```python
from build123d import *

# Parameters (mm, degrees)
F0_R     = 12.7
F1_DEPTH = 44.45
F2_W     = 127
F2_H     = 67.31
F3_DEPTH = 12.7
F4_R     = 5.08
F5_DEPTH = 13.7612578348


with BuildPart() as f1:
    # F0 (on Front) → F1 (new body)
    with BuildSketch(Plane.XZ):
        with BuildLine():
            Line((-31.75, 12.7), (-31.75, 0))
            Line((-31.75, 0), (31.75, 0))
            Line((31.75, 0), (31.75, 12.7))
            Line((31.75, 12.7), (12.7, 12.7))
            Line((12.7, 12.7), (12.7, 21.59))
            Line((12.7, 21.59), (63.5, 21.59))
            Line((63.5, 21.59), (63.5, 34.29))
            Line((63.5, 34.29), (47.625, 34.29))
            Line((47.625, 34.29), (21.6717633531, 76.7474402496))
            ThreePointArc((21.6717633531, 76.7474402496), (0, 88.9), (-21.6717633531, 76.7474402496))
            Line((-21.6717633531, 76.7474402496), (-47.625, 34.29))
            Line((-47.625, 34.29), (-63.5, 34.29))
            Line((-63.5, 34.29), (-63.5, 21.59))
            Line((-63.5, 21.59), (-12.7, 21.59))
            Line((-12.7, 21.59), (-12.7, 12.7))
            Line((-12.7, 12.7), (-31.75, 12.7))
        make_face()
        with Locations((0, 63.5)):
            Circle(F0_R, mode=Mode.SUBTRACT)
    extrude(amount=F1_DEPTH)

    # F2 (on face) → F3 (join)
    with BuildSketch(Plane(origin=(0, 0, 0), x_dir=(-1, 0, 0), z_dir=(0, 1, 0))):
        with Locations((0, 55.245)):
            Rectangle(F2_W, F2_H)
        Polygon((12.7, 21.59), (-12.7, 21.59), (-12.7, 12.7), (-31.75, 12.7), (-31.75, 0), (31.75, 0), (31.75, 12.7), (12.7, 12.7), align=None)
    extrude(amount=F3_DEPTH)

    # F4 (on face) → F5 (cut, through all)
    with BuildSketch(Plane.XY.offset(88.9)):
        with Locations((0, -22.225)):
            Circle(F4_R)
    extrude(amount=-F5_DEPTH, mode=Mode.SUBTRACT)


solid = f1.part
```
Source: CAD feature listing. Evaluate the final solid. Frame: model axes, mm. A direction names the side the tool comes from. Coordinates: 2 decimals unless noted, no trailing zeros. Order: outer loops, then holes, each group sorted by start corner. A loop starts at its lowest first (then second) coordinate and runs counter-clockwise, first axis right, second up. Notation, with made-up numbers: M -36.75,9 L 18.25,9 A26 ccw 18.25,43 Z; hole C 47.5,73.25 d3. An arc over 180 degrees is marked long. Write each question's results on one line, items separated by ' | '. Start each with the question number.
1) Section query A-A (y = -34). Return the cut outline in (x, z) (3 decimals), plus the area to 3 significant figures.
2) Draft query along X for faces 6 (the face through (1, 12.7, 55)), 7 (the face through (5.86, -21.914, 52.233)), 8 (the face through (0.363, -16.975, 88.897)). Return one class per face: released by +X, released by -X, zero draft, split by the parting line, or undercut.
3) Contact query for flat-ended pins moving along their axis: pin 1 Ø1.5 at (x, y) = (47, 0) entering from -Z; pin 2 Ø6.5 at (y, z) = (-18.5, 6) entering from +X; pin 3 Ø15 at (x, y) = (-24.5, -27.5) entering from +Z. Output: stop coordinate, or through.
4) Section query D-D (x = 55). Return the cut outline in (y, z).
5) Section query B-B (x = 20). Return the cut outline in (y, z), plus the area to 3 significant figures.
6) Line query: line 1 (Z direction, x = 0, y = -10.5); line 2 (Y direction, x = 0, z = 80.75) (3 decimals); line 3 (Y direction, x = -53.5, z = 60.5). Output: solid intervals per line, ascending. Write a range as from..to.
7) Access query for faces 1 (the face through (46, 0, 68)), 2 (the face through (0, 0, 64)), 3 (the face through (-38, -16, 21.59)), 4 (the face through (-34.467, -21.914, 55.816)), 5 (the face through (-31.75, -16, 6)). Directions: +Z, -Z, +X, -X, +Y, -Y. A direction counts if a zero-diameter tool reaches every point of the face in a straight line with its end or side. Return the directions, or none.
8) Section query C-C (z = 44.5). Return the cut outline in (x, y), plus the area to 3 significant figures.
Answers:
1) outline: M -63.5,21.59 L -12.7,21.59 L -12.7,12.7 L -31.75,12.7 L -31.75,0 L 31.75,0 L 31.75,12.7 L 12.7,12.7 L 12.7,21.59 L 63.5,21.59 L 63.5,34.29 L 47.625,34.29 L 21.672,76.747 A25.4 ccw -21.672,76.747 L -47.625,34.29 L -63.5,34.29 Z; hole C 0,63.5 d25.4 | area: 5,450 mm^2
2) face 6: zero draft | face 7: undercut | face 8: split by the parting line
3) pin 1: stops at z = 21.59 | pin 2: stops at x = 31.75 | pin 3: stops at z = 82.37
4) outline: M -44.45,21.59 L 12.7,21.59 L 12.7,88.9 L 0,88.9 L 0,34.29 L -44.45,34.29 Z
5) outline: M -44.45,0 L 12.7,0 L 12.7,12.7 L -44.45,12.7 Z; M -44.45,21.59 L 12.7,21.59 L 12.7,88.9 L 0,88.9 L 0,79.16 L -44.45,79.16 Z | area: 4,140 mm^2
6) line 1: z = 0..50.8, 76.2..88.9 | line 2: y = -44.45..-27.305, -17.145..12.7 | line 3: y = 0..12.7
7) face 1: +Z, +X, -Y | face 2: -Y | face 3: -X, +Y, -Y | face 4: +Z, -X, -Y | face 5: -Z, -X, +Y, -Y
8) outline: M -63.5,0 L -41.38,0 L -41.38,-44.45 L 41.38,-44.45 L 41.38,0 L 63.5,0 L 63.5,12.7 L -63.5,12.7 Z | area: 5,290 mm^2
